Here's how the part is built. I have some questions about the finished solid (model axes, mm). Round coordinates to 2 decimals unless told otherwise and drop trailing zeros. Order: outer loops, then holes, each group sorted by start corner. A loop starts at its lowest first (then second) coordinate and runs counter-clockwise, first axis right, second up. Notation, with made-up numbers: M 22,2 L 51,2 A30 ccw 51,41 Z; hole C -5,-17.5 d3. An arc over 180 degrees is marked long. Write item = value, one per line. Start each with the question number.
Item 1: I want a section at B-B, the plane z = 0. List the corners of the cut face in (x, y) for me, plus the area to 4 significant figures.
Item 2: We'd pull the mould along X, two halves only. Please class faces 1 (the face through (-2.777, -0.74, 6.697)), 2 (the face through (-20, -1, 0)), 3 (the face through (20, -1, 0)): pulls with the +X half, pulls with the -X half, needs draft (parallel to the pull), parting line crosses it, or undercut.
Item 3: I want a section at D-D, the plane x = 0. List the corners of the cut face in (y, z) for me.
Item 4: I want a section at A-A, the plane x = -5. List the corners of the cut face in (y, z) for me.
Item 5: I want a section at C-C, the plane y = -0.4. List the corners of the cut face in (x, z) for me.
Item 6: Please list where these lines run through material, in increasing order: L1, parallel to X at y = -0.85, z = 20; L2, parallel to X at y = -1, z = 0; L3, parallel to Z at x = 4, y = -1.4.
```python
from build123d import *

# Parameters (mm, degrees)
ESQUISSE1_W               = 40
ESQUISSE1_H               = 65
T_LE_DE_BASE_PLI_E1_DEPTH = 1.5
PASSAGE_VIS_M5_REACH      = 40.19
ESQUISSE6_R               = 2.6
PASSAGE_JAUGE_REACH       = 40.19
ESQUISSE7_R               = 7.25


# Sheet-metal steps are written as plain solids
with BuildPart() as part:
    # Esquisse1 → Tôle de base pliée1 (new body)
    with BuildSketch(Plane(origin=(0, 0, 0), x_dir=(1, 0, 0), z_dir=(0, 1, 0))):
        Rectangle(ESQUISSE1_W, ESQUISSE1_H)
    extrude(amount=-T_LE_DE_BASE_PLI_E1_DEPTH)

    # Esquisse6 → Passage_Vis_M5 (cut, up to next)
    with BuildSketch(Plane(origin=(0, 0, 0), x_dir=(1, 0, 0), z_dir=(0, 1, 0)), mode=Mode.PRIVATE) as passage_vis_m5_sk1:
        with Locations(Location((0, 20, 0), (0, 0, 270))):
            Circle(ESQUISSE6_R)
    passage_vis_m5_tool1 = extrude(passage_vis_m5_sk1.sketch, amount=-PASSAGE_VIS_M5_REACH, mode=Mode.PRIVATE) & part.part
    # Esquisse6 → Passage_Vis_M5 (cut, up to next)
    with BuildSketch(Plane(origin=(0, 0, 0), x_dir=(1, 0, 0), z_dir=(0, 1, 0)), mode=Mode.PRIVATE) as passage_vis_m5_sk2:
        with Locations(Location((0, -20, 0), (0, 0, 90))):
            Circle(ESQUISSE6_R)
    passage_vis_m5_tool2 = extrude(passage_vis_m5_sk2.sketch, amount=-PASSAGE_VIS_M5_REACH, mode=Mode.PRIVATE) & part.part
    add(passage_vis_m5_tool1.solids().sort_by_distance((0, 0, -20))[0], mode=Mode.SUBTRACT)
    add(passage_vis_m5_tool2.solids().sort_by_distance((0, 0, 20))[0], mode=Mode.SUBTRACT)

    # Esquisse7 → Passage_Jauge (cut, up to next)
    with BuildSketch(Plane(origin=(0, 0, 0), x_dir=(1, 0, 0), z_dir=(0, 1, 0)), mode=Mode.PRIVATE) as passage_jauge_sk1:
        with Locations(Location((0, 0, 0), (0, 0, 270))):
            Circle(ESQUISSE7_R)
    passage_jauge_tool1 = extrude(passage_jauge_sk1.sketch, amount=-PASSAGE_JAUGE_REACH, mode=Mode.PRIVATE) & part.part
    add(passage_jauge_tool1.solids().sort_by_distance((0, 0, 0))[0], mode=Mode.SUBTRACT)


solid = part.part
```
Filled in:
q1.outline = M -20,-1.5 L -7.25,-1.5 L -7.25,0 L -20,0 Z; M 7.25,-1.5 L 20,-1.5 L 20,0 L 7.25,0 Z
q1.area = 38.25 mm^2
q2.face_1 = undercut
q2.face_2 = pulls with the -X half
q2.face_3 = pulls with the +X half
q3.outline = M -1.5,-32.5 L 0,-32.5 L 0,-22.6 L -1.5,-22.6 Z; M -1.5,-17.4 L 0,-17.4 L 0,-7.25 L -1.5,-7.25 Z; M -1.5,7.25 L 0,7.25 L 0,17.4 L -1.5,17.4 Z; M -1.5,22.6 L 0,22.6 L 0,32.5 L -1.5,32.5 Z
q4.outline = M -1.5,-32.5 L 0,-32.5 L 0,-5.25 L -1.5,-5.25 Z; M -1.5,5.25 L 0,5.25 L 0,32.5 L -1.5,32.5 Z
q5.outline = M -20,-32.5 L 20,-32.5 L 20,32.5 L -20,32.5 Z; hole C 0,0 d14.5; hole C 0,-20 d5.2; hole C 0,20 d5.2
q6.L1 = -20 to -2.6, 2.6 to 20
q6.L2 = -20 to -7.25, 7.25 to 20
q6.L3 = -32.5 to -6.05, 6.05 to 32.5
